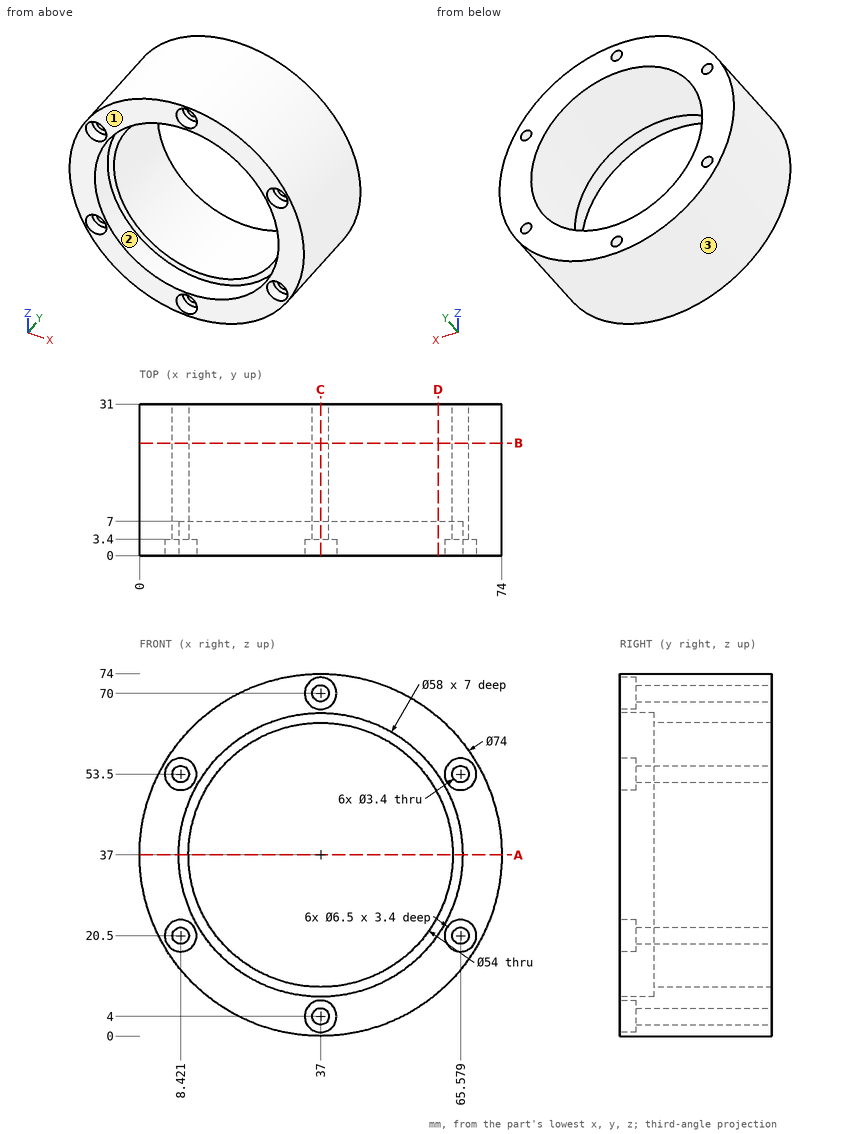
The figure shows three views and two pictorial views of one solid part (mm, origin at its lowest corner). Answer the questions. Coordinates: 2 decimals unless noted, no trailing zeros. Loops run counter-clockwise (first coordinate to the right, second up) from the corner with the lowest first, then second, coordinate; pieces in that order, holes last.
(1) The part is cut by section A-A (z = 37). Determine the outline of the cut face in (x, y), and give its area (3 significant figures).
Solution:
outline: (0, 0) - (8, 0) - (8, 7) - (10, 7) - (10, 31) - (0, 31) - close; (64, 7) - (66, 7) - (66, 0) - (74, 0) - (74, 31) - (64, 31) - close
area: 592 mm2
(2) Flat-ended cylindrical pins translate along their axes: pin 1 Ø3 at (x, z) = (11.5, 48) entering from -Y; pin 2 Ø6 at (x, z) = (65.58, 20.5) entering from -Y; pin 3 Ø6 at (y, z) = (14.5, 22) entering from -X; pin 4 Ø12 at (y, z) = (5, 18) entering from +X. Find the tip coordinate at first contact, or state that the pin passes through.
Solution:
pin 1: stops at y = 0
pin 2: stops at y = 3.4
pin 3: stops at x = 2
pin 4: stops at x = 71.64
(3) The mould has two halves that part along Z. Classify the marked faces 1, 2 and 3: released by +Z, released by -Z, zero draft, split by the parting line, or undercut.
Solution:
face 1: zero draft
face 2: undercut
face 3: split by the parting line
(4) The part is cut by section C-C (x = 37). Determine the outline of the cut face in (y, z), and give its area (3 significant figures).
Solution:
outline: (0, 0) - (31, 0) - (31, 2.3) - (3.4, 2.3) - (3.4, 0.75) - (0, 0.75) - close; (0, 7.25) - (3.4, 7.25) - (3.4, 5.7) - (31, 5.7) - (31, 10) - (7, 10) - (7, 8) - (0, 8) - close; (0, 66) - (7, 66) - (7, 64) - (31, 64) - (31, 68.3) - (3.4, 68.3) - (3.4, 66.75) - (0, 66.75) - close; (0, 73.25) - (3.4, 73.25) - (3.4, 71.7) - (31, 71.7) - (31, 74) - (0, 74) - close
area: 360 mm2
(5) Consider line 1 along Y through (x, z) = (19.5, 15); line 2 along X through (y, z) = (26.5, 46.5); line 3 along X through (y, z) = (17, 4). Determine where each line is inside the solid, lowest interval first.
Solution:
line 1: y = 7 to 31
line 2: x = 1.24 to 11.73, 62.27 to 72.76
line 3: x = 20.27 to 35.3, 38.7 to 53.73
(6) The part is cut by section D-D (x = 61). Determine the outline of the cut face in (y, z), and give its area (3 significant figures).
Solution:
outline: (0, 8.84) - (31, 8.84) - (31, 24.63) - (7, 24.63) - (7, 20.72) - (0, 20.72) - close; (0, 53.28) - (7, 53.28) - (7, 49.37) - (31, 49.37) - (31, 65.16) - (0, 65.16) - close
area: 924 mm2
(7) The part is cut by section B-B (y = 23). Determine the outline of the cut face in (x, z), and give its area (3 significant figures).
Solution:
outline: circle Ø74 at (37, 37); hole circle Ø3.4 at (8.42, 20.5); hole circle Ø3.4 at (8.42, 53.5); hole circle Ø54 at (37, 37); hole circle Ø3.4 at (37, 4); hole circle Ø3.4 at (37, 70); hole circle Ø3.4 at (65.58, 20.5); hole circle Ø3.4 at (65.58, 53.5)
area: 1,960 mm2
